Here's how the part is built. I have some questions about the finished solid (model axes, mm). A direction names the side the tool comes from. Coordinates: 2 decimals unless noted, no trailing zeros. Write each loop counter-clockwise with the first axis right and the second up, starting at its lowest first coordinate (ties: lowest second). Pieces come first, ordered by that corner, then holes.
(1) Imagine slicing it at B-B, the plane z = 9. List the corners of the cut face in (x, y) for me, plus the area to 3 significant figures.
(2) Thinking about a two-plate mould opening in Y: for faces 5 (the flat face through (1.7, 4.5, 1)), 6 (the flat face through (1.3, 10, 9)), 7 (the flat face through (-2.8, 16.2, 1.1)), which applies, released by +Y, released by -Y, zero draft, split by the parting line, or undercut?
(3) Which directions (+Z, -Z, +X, -X, +Y, -Y) give clear straight access to the entire face, cutting with the end or side of a thin tool? Please do faces 1 (the flat face through (1.7, 12.5, 17)), 2 (the flat face through (-1, 4.5, 17)), 3 (the flat face through (-1, 4.5, 1)), 4 (the flat face through (-2.514, 9.071, 11.586)).
(4) Imagine slicing it at C-C, the plane x = -0.25. List the corners of the cut face in (y, z) for me, plus the area to 3 significant figures.
(5) For pin 1 Ø5.5 at (y, z) = (7.55, 9) entering from -X; pin 2 Ø0.6 at (x, z) = (1.5, 12) entering from +Y; pin 3 Ø0.7 at (x, z) = (-1.5, 12.5) entering from -Y, each with a flat end and sliding along its axis, tell me the tip position at first contact or that it passes through.
(6) Imagine slicing it at D-D, the plane z = 16.5. List the corners of the cut face in (x, y) for me, plus the area to 3 significant figures.
(7) Imagine slicing it at A-A, the plane y = -0.25. List the corners of the cut face in (x, z) for me.
(8) Please list where these lines run through material, in increasing order: probe 1 along X at (y, z) = (2, 6.75); probe 2 along Y at (x, z) = (-0.3, 9); probe 3 along X at (y, z) = (8.5, 12.25).
Autodesk Fusion 360 part; units mm, degrees
sketch "Sketch1" plane through (0, 0, 0) normal (0, 0, 1) x (1, 0, 0)
  line L0 (1.75, -1.4) -> (1.75, 1.4) construction
  arc A0 (1.75, 1.4) -> (-1.75, 1.4) centre (0, 1.4) ccw construction
  line L1 (-1.75, 1.4) -> (-1.75, -1.4) construction
  arc A1 (-1.75, -1.4) -> (1.75, -1.4) centre (0, -1.4) ccw construction
  line L2 (0, -1.4) -> (0, 1.4) construction
  line L3 (0, 3.15) -> (0, -3.15) construction
  line L4 (-2.1, 19.1) -> (-2.1, -1.4)
  arc A2 (-2.1, -1.4) -> (2.1, -1.4) centre (0, -1.4) ccw
  line L5 (2.1, -1.4) -> (2.1, 19.1)
  line L6 (-2.1, 19.1) -> (-3.5, 19.1)
  line L7 (-3.5, 19.1) -> (-3.5, -1.4)
  line L8 (2.1, 19.1) -> (3.5, 19.1)
  line L9 (3.5, 19.1) -> (3.5, -1.4)
  arc A3 (-3.5, -1.4) -> (3.5, -1.4) centre (0, -1.4) ccw
  line L10 (2.1, 13.5) -> (1.3, 13.5)
  line L11 (1.3, 13.5) -> (1.3, 3.5)
  line L12 (1.3, 3.5) -> (2.1, 3.5)
  line L13 (-2.1, 13.5) -> (0.1, 13.5)
  line L14 (0.1, 13.5) -> (0.1, 3.5)
  line L15 (0.1, 3.5) -> (-2.1, 3.5)
  point P0 (0, -4.9)
  dimension "d1" = 3.5
  dimension "d2" = 6.3
  dimension "d12" = 24
  dimension "d14" = 2.1
  dimension "d15" = 1.4
  dimension "d16" = 10
  dimension "d17" = 3.5
  dimension "d25" = 2.2
  dimension "d26" = 0.8
extrude "Extrude1" add sketch "Sketch1" along normal blind 18
sketch "Sketch2" plane through (0, 0, 0) normal (1, 0, 0) x (0, 1, 0)
  line L0 (19.1, 0) -> (19.1, 18)
  circle A0 centre (7.55, 9) radius 1.75
  line L1 (3.15, 0) -> (1.4, 0)
  line L2 (7.55, 9) -> (5.8, 9) construction
  line L3 (10.55, 10.7321) -> (7.55, 12.4641)
  line L4 (7.55, 12.4641) -> (4.55, 10.7321)
  line L5 (4.55, 10.7321) -> (4.55, 7.2679)
  line L6 (4.55, 7.2679) -> (7.55, 5.5359)
  line L7 (7.55, 5.5359) -> (10.55, 7.2679)
  line L8 (10.55, 7.2679) -> (10.55, 10.7321)
  point P0 (19.1, 9)
  point P1 (3.15, 0)
  point P2 (7.55, 9)
  dimension "d7" = 3.5
  dimension "d20" = 6
  dimension "d24" = 1.4
extrude "Extrude2" cut sketch "Sketch2" along normal mid plane 14 contours A0
chamfer "Chamfer1" distance 4 angle 45 4 edges at (2.8, 19.1, 0) (-2.8, 19.1, 0) (2.8, 19.1, 18) (-2.8, 19.1, 18)
fillet "Fillet1" radius 6 4 edges at (2.8, 19.1, 4) (2.8, 19.1, 14) (-2.8, 19.1, 4) (-2.8, 19.1, 14)
extrude "Extrude3" cut sketch "Sketch2" along normal blind 2 from surface at -3.5
chamfer "Chamfer2" distance 2 angle 45 8 edges at (-1, 13.5, 18) (-1, 3.5, 18) (1.7, 13.5, 18) (1.7, 3.5, 18) (1.7, 13.5, 0) (-1, 13.5, 0) (1.7, 3.5, 0) (-1, 3.5, 0)
Recorded:
1. outline: (-3.5, -1.4) arc R3.5 ccw to (3.5, -1.4) - (3.5, 5.8) - (1.3, 5.8) - (1.3, 3.5) - (2.1, 3.5) - (2.1, -1.4) arc R2.1 cw to (-2.1, -1.4) - (-2.1, 3.5) - (0.1, 3.5) - (0.1, 5.8) - (-1.5, 5.8) - (-1.5, 4.55) - (-3.5, 4.55) - close; (-3.5, 10.55) - (-1.5, 10.55) - (-1.5, 9.3) - (0.1, 9.3) - (0.1, 13.5) - (-2.1, 13.5) - (-2.1, 19.1) - (-3.5, 19.1) - close; (1.3, 9.3) - (3.5, 9.3) - (3.5, 19.1) - (2.1, 19.1) - (2.1, 13.5) - (1.3, 13.5) - close
1. area: 74.4 mm2
2. face 5: undercut
2. face 6: zero draft
2. face 7: released by +Y
3. face 1: +Z, +Y
3. face 2: +Z
3. face 3: -Z
3. face 4: -X
4. outline: (-4.89, 0) - (-3.49, 0) - (-3.49, 18) - (-4.89, 18) - close; (3.5, 2) - (5.5, 0) - (11.5, 0) - (13.5, 2) - (13.5, 16) - (11.5, 18) - (5.5, 18) - (3.5, 16) - close; hole circle Ø3.5 at (7.55, 9)
4. area: 188 mm2
5. pin 1: stops at x = -1.5
5. pin 2: stops at y = 13.5
5. pin 3: stops at y = -4.71
6. outline: (-3.5, -1.4) arc R3.5 ccw to (3.5, -1.4) - (3.5, 16.6) - (2.1, 16.6) - (2.1, 13) - (1.3, 13) - (1.3, 4) - (2.1, 4) - (2.1, -1.4) arc R2.1 cw to (-2.1, -1.4) - (-2.1, 4) - (0.1, 4) - (0.1, 13) - (-2.1, 13) - (-2.1, 16.6) - (-3.5, 16.6) - close
6. area: 89.7 mm2
7. outline: (-3.5, 0) - (-2.1, 0) - (-2.1, 18) - (-3.5, 18) - close; (2.1, 0) - (3.5, 0) - (3.5, 18) - (2.1, 18) - close
8. probe 1: x = -3.5 to -2.1, 2.1 to 3.5
8. probe 2: y = -4.89 to -3.48, 3.5 to 5.8, 9.3 to 13.5
8. probe 3: x = -3.5 to 0.1, 1.3 to 3.5
